Answer from the drawing. Dimensions are ordinates in mm from the lowest x, y and z of the part. Coordinates: 2 decimals unless noted, no trailing zeros. Write each loop counter-clockwise with the first axis right and the second up, starting at its lowest first coordinate (ties: lowest second). Pieces come first, ordered by that corner, then holes. Notation, with made-up numbers: (78.5, -6) -> (123.5, -6) arc R21 cw to (123.5, 5) -> close; hole circle Ø10 at (-8.5, 84). An arc over 180 degrees is marked (long way). Answer as a JSON object with one key per item and string values. Group by question number.
(1) Find section B-B (y = 1.2). Give the vertices of the cut face in (x, z), then the cut area to 3 significant figures.
(2) Find section C-C (z = 60). Give the vertices of the cut face in (x, y), then the cut area to 3 significant figures.
(3) Flat-ended cylindrical pins translate along their axes: P1, Ø1, axis at x = 61.5, y = 2.5, coming from the +Z side; P2, Ø2, axis at y = 3.5, z = 55.5, coming from the -X side; P3, Ø1.5, axis at x = 76.5, y = 2, coming from the -Z side. Find the tip coordinate at first contact, or state that the pin passes through.
(4) Straight lines are drawn through the part: L1, parallel to X at y = 3.75, z = 60; L2, parallel to Z at x = 61, y = 0.95; L3, parallel to X at y = 1.8, z = 52. For each, find the intervals that lie inside material, in ascending order.
(5) Find section D-D (x = 105). Give the vertices of the cut face in (y, z).
(6) Find section A-A (x = 60). Give the vertices of the cut face in (y, z), then the cut area to 3 significant figures.
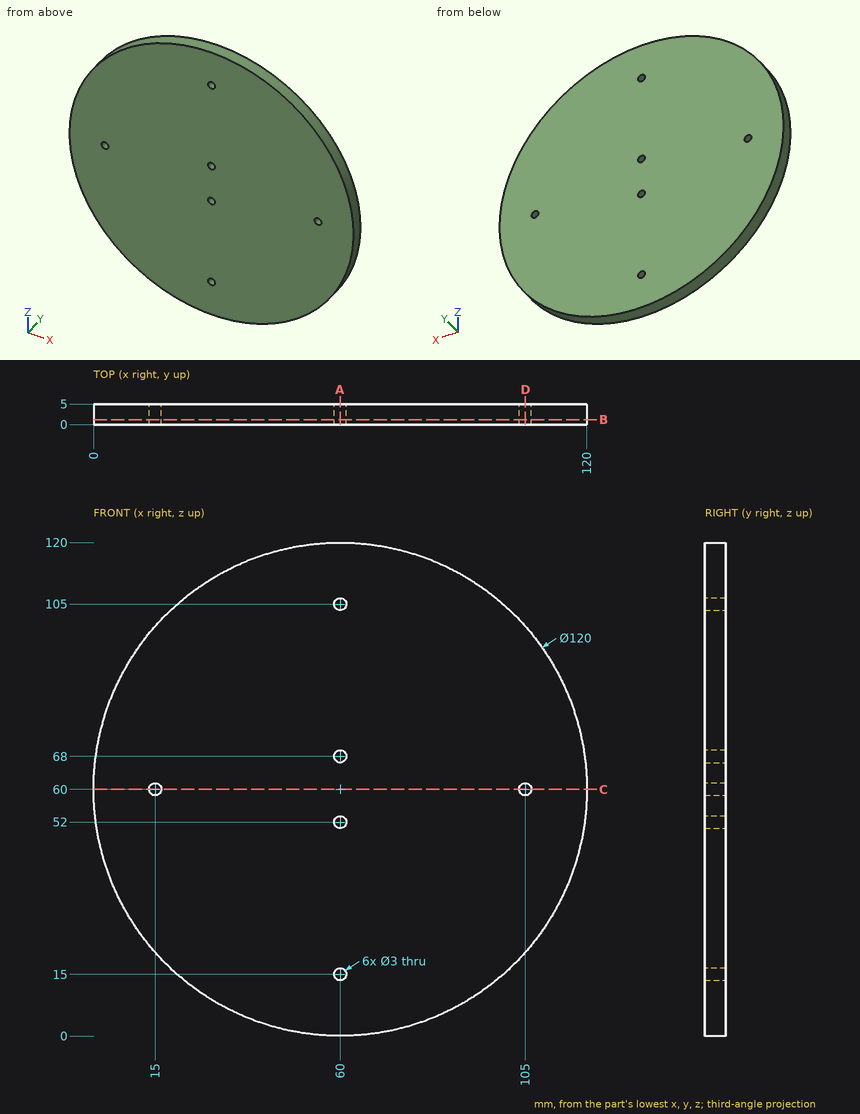
Results below:
{
 "1": {"outline": "circle Ø120 at (60, 60); hole circle Ø3 at (15, 60); hole circle Ø3 at (60, 15); hole circle Ø3 at (60, 52); hole circle Ø3 at (60, 68); hole circle Ø3 at (60, 105); hole circle Ø3 at (105, 60)", "area": "11,300 mm2"},
 "2": {"outline": "(0, 0) -> (13.5, 0) -> (13.5, 5) -> (0, 5) -> close; (16.5, 0) -> (103.5, 0) -> (103.5, 5) -> (16.5, 5) -> close; (106.5, 0) -> (120, 0) -> (120, 5) -> (106.5, 5) -> close", "area": "570 mm2"},
 "3": {"P1": "stops at z = 119.99", "P2": "stops at x = 0.1", "P3": "stops at z = 2.1"},
 "4": {"L1": "x = 0 to 13.5, 16.5 to 103.5, 106.5 to 120", "L2": "z = 0.01 to 13.88, 16.12 to 50.88, 53.12 to 66.88, 69.12 to 103.88, 106.12 to 119.99", "L3": "x = 0.54 to 58.5, 61.5 to 119.46"},
 "5": {"outline": "(0, 20.31) -> (5, 20.31) -> (5, 58.5) -> (0, 58.5) -> close; (0, 61.5) -> (5, 61.5) -> (5, 99.69) -> (0, 99.69) -> close"},
 "6": {"outline": "(0, 0) -> (5, 0) -> (5, 13.5) -> (0, 13.5) -> close; (0, 16.5) -> (5, 16.5) -> (5, 50.5) -> (0, 50.5) -> close; (0, 53.5) -> (5, 53.5) -> (5, 66.5) -> (0, 66.5) -> close; (0, 69.5) -> (5, 69.5) -> (5, 103.5) -> (0, 103.5) -> close; (0, 106.5) -> (5, 106.5) -> (5, 120) -> (0, 120) -> close", "area": "540 mm2"}
}
